from build123d import *

# Parameters (mm, degrees)
SKETCH1_W                    = 25
SKETCH1_H                    = 35
SKETCH1_R                    = 4.5
SKETCH1_R_2                  = 2
BASE_FLANGE1_DEPTH           = 1.5
EDGE_FLANGE1_STRIP_W         = 7.4732
EDGE_FLANGE1_STRIP_H         = 1.5
EDGE_FLANGE1_STRIP_CUT_DEPTH = 25
EDGE_FLANGE1_DEPTH           = 25
SKETCH9_R                    = 4.5
SKETCH9_R_2                  = 2
CUT_EXTRUDE1_DEPTH           = 10
FILLET1_R                    = 12.5


# Sheet-metal steps are written as plain solids
with BuildPart() as part:
    # Sketch1 → Base-Flange1 (new body)
    with BuildSketch(Plane(origin=(0, 0, 0), x_dir=(1, 0, 0), z_dir=(0, 1, 0))):
        Rectangle(SKETCH1_W, SKETCH1_H)
        with Locations(Location((0, -5.5, 0), (0, 0, 270))):
            Circle(SKETCH1_R, mode=Mode.SUBTRACT)
        with Locations(Location((-7, -5.5, 0), (0, 0, 270))):
            Circle(SKETCH1_R_2, mode=Mode.SUBTRACT)
        with Locations(Location((0, -12.5, 0), (0, 0, 270))):
            Circle(SKETCH1_R_2, mode=Mode.SUBTRACT)
        with Locations(Location((7, -5.5, 0), (0, 0, 270))):
            Circle(SKETCH1_R_2, mode=Mode.SUBTRACT)
        with Locations(Location((0, 1.5, 0), (0, 0, 270))):
            Circle(SKETCH1_R_2, mode=Mode.SUBTRACT)
    extrude(amount=BASE_FLANGE1_DEPTH)

    # Edge-Flange1 strip (across the edge) → Edge-Flange1 strip cut (cut)
    with BuildSketch(Plane(origin=(12.5, 1.5, -17.5), x_dir=(0, 0, 1), z_dir=(-1, 0, 0))):
        with Locations((-1.5, -0.75)):
            Rectangle(EDGE_FLANGE1_STRIP_W, EDGE_FLANGE1_STRIP_H)
    extrude(amount=EDGE_FLANGE1_STRIP_CUT_DEPTH, mode=Mode.SUBTRACT)

    # Edge-Flange1 section (across the edge) → Edge-Flange1 (add)
    with BuildSketch(Plane(origin=(12.5, 1.5, -17.5), x_dir=(0, 0, 1), z_dir=(-1, 0, 0))):
        with BuildLine():
            Line((0, 0.7366), (0, 28))
            Line((0, 28), (1.5, 28))
            Line((1.5, 28), (1.5, 0.7366))
            ThreePointArc((1.5, 0.7366), (1.715745145, 0.215745145), (2.2366, 0))
            Line((2.2366, 0), (2.2366, -1.5))
            ThreePointArc((2.2366, -1.5), (0.655084973, -0.844915027), (0, 0.7366))
        make_face()
    extrude(amount=EDGE_FLANGE1_DEPTH)

    # Sketch9 → Cut-Extrude1 (cut)
    with BuildSketch(Plane.XY.offset(-16)):
        with Locations((0, 17)):
            Circle(SKETCH9_R)
        with Locations((-7, 17)):
            Circle(SKETCH9_R_2)
        with Locations((7, 17)):
            Circle(SKETCH9_R_2)
        with Locations((0, 24)):
            Circle(SKETCH9_R_2)
        with Locations((0, 10)):
            Circle(SKETCH9_R_2)
    extrude(amount=-CUT_EXTRUDE1_DEPTH, mode=Mode.SUBTRACT)

    # Fillet1
    fillet1_edges = [part.edges().sort_by_distance(p)[0] for p in [
        (12.5, 0.75, 17.5),
        (-12.5, 0.75, 17.5),
        (12.5, 29.5, -16.75),
        (-12.5, 29.5, -16.75),
    ]]
    fillet(fillet1_edges, radius=FILLET1_R - 0.0001)  # a hair under: the kernel refuses the full size


solid = part.part
Source: CAD feature listing. Evaluate the final solid. Frame: model axes, mm. A direction names the side the tool comes from. Coordinates: 2 decimals unless noted, no trailing zeros. Loops run counter-clockwise (first coordinate to the right, second up) from the corner with the lowest first, then second, coordinate; pieces in that order, holes last. Notation, with made-up numbers: M 83,30.25 L 91,30.25 A24 ccw 91,54.25 Z; hole C -36,47 d8. An arc over 180 degrees is marked long. Answer in a Markdown table with one row per item.
Q1. Set-up query: faces 4 (the cylindrical face through (-1.2, 0.7, 10.9)), 5 (the flat face through (-3, 13, -16)). Return all of +Z, -Z, +X, -X, +Y, -Y with unobstructed straight access to the full face (end or side cutting, diameter ignored); none if empty.
Answers below:
| item | result |
|---|---|
| face 4 | +Y, -Y |
| face 5 | +Z, +X, -X, +Y |
Q2. Ray query, probe 1 along X at (y, z) = (0.4, 5.5); probe 2 along X at (y, z) = (1.15, -1.5); probe 3 along Y at (x, z) = (-10.25, 0.5). Return the intervals inside material, ascending. Write a range as from..to.
Answers below:
| item | result |
|---|---|
| probe 1 | x = -12.49..-9, -5..-4.5, 4.5..5, 9..12.49 |
| probe 2 | x = -12.5..-2, 2..12.5 |
| probe 3 | y = 0..1.5 |
Q3. Section A-A on z = -1.5. Return the cut outline in (x, y), plus the area to 3 significant figures.
Answers below:
| item | result |
|---|---|
| outline | M -12.5,0 L -2,0 L -2,1.5 L -12.5,1.5 Z; M 2,0 L 12.5,0 L 12.5,1.5 L 2,1.5 Z |
| area | 31.5 mm^2 |
Q4. First-contact query: pin 1 (2 mm diameter, centred on x = 9.5, y = 8.5, fed in from +Z); pin 2 (4.5 mm diameter, centred on x = 0, z = -1.5, fed in from +Y). Flat tips, straight axial feed; report the tip coordinate or a pass-through.
Answers below:
| item | result |
|---|---|
| pin 1 | stops at z = -16 |
| pin 2 | stops at y = 1.5 |
Q5. Section C-C on z = 7. Return the cut outline in (x, y).
Answers below:
| item | result |
|---|---|
| outline | M -12.34,0 L -8.32,0 L -8.32,1.5 L -12.34,1.5 Z; M -5.68,0 L -4.24,0 L -4.24,1.5 L -5.68,1.5 Z; M 4.24,0 L 5.68,0 L 5.68,1.5 L 4.24,1.5 Z; M 8.32,0 L 12.34,0 L 12.34,1.5 L 8.32,1.5 Z |
Q6. Draft query along Y for faces 1 (the cylindrical face through (1.352, 0.74, 9.792)), 2 (the flat face through (-3, 1.5, -3)), 3 (the cylindrical face through (0, 12, -17)). Return one class per face: pulls with the +Y half, pulls with the -Y half, needs draft (parallel to the pull), parting line crosses it, or undercut.
Answers below:
| item | result |
|---|---|
| face 1 | needs draft |
| face 2 | pulls with the +Y half |
| face 3 | undercut |
Q7. Section B-B on x = -2.5. Return the cut outline in (y, z), plus the area to 3 significant figures.
Answers below:
| item | result |
|---|---|
| outline | M 0,-15.26 A2.24 ccw 2.24,-17.5 L 13.26,-17.5 L 13.26,-16 L 2.24,-16 A0.74 cw 1.5,-15.26 L 1.5,1.76 L 0,1.76 Z; M 0,9.24 L 1.5,9.24 L 1.5,17.25 L 0,17.25 Z; M 20.74,-17.5 L 29.25,-17.5 L 29.25,-16 L 20.74,-16 Z |
| area | 70.3 mm^2 |
Q8. Section D-D on y = 24. Return the cut outline in (x, z).
Answers below:
| item | result |
|---|---|
| outline | M -10.36,-17.5 L -2,-17.5 L -2,-16 L -10.36,-16 Z; M 2,-17.5 L 10.36,-17.5 L 10.36,-16 L 2,-16 Z |
